Geometry: final body of the model. Coordinates: model frame, mm. A direction names the side the tool comes from. Round coordinates to 2 decimals unless told otherwise and drop trailing zeros. Order: outer loops, then holes, each group sorted by start corner. A loop starts at its lowest first (then second) coordinate and runs counter-clockwise, first axis right, second up. Notation, with made-up numbers: (-9, -27.5) -> (0, -27.5) arc R23 ccw to (0, -3.5) -> close; hole circle Ø5 at (64, 50.25). An arc over 180 degrees is marked (long way). Put each result on its own line as item: value.
```python
from build123d import *


with BuildPart() as part:
    # Sketch1 → Revolve1 (revolve)
    with BuildSketch(Plane.XY, mode=Mode.PRIVATE) as revolve1_sk:
        with BuildLine():
            Line((0, 0), (0, 10))
            Line((0, 10), (15, 10))
            Line((15, 10), (15, 15))
            Line((15, 15), (20, 15))
            ThreePointArc((20, 15), (27.5, 12.990381057), (32.990381057, 7.5))
            Line((32.990381057, 7.5), (35.990381057, 7.5))
            Line((35.990381057, 7.5), (37.490381057, 10))
            Line((37.490381057, 10), (40.490381057, 10))
            Line((40.490381057, 10), (41.990381057, 7.5))
            Line((41.990381057, 7.5), (44.990381057, 7.5))
            Line((44.990381057, 7.5), (46.490381057, 10))
            Line((46.490381057, 10), (49.490381057, 10))
            Line((49.490381057, 10), (50.990381057, 7.5))
            Line((50.990381057, 7.5), (53.990381057, 7.5))
            Line((53.990381057, 7.5), (55.490381057, 10))
            Line((55.490381057, 10), (58.490381057, 10))
            Line((58.490381057, 10), (59.990381057, 7.5))
            Line((59.990381057, 7.5), (62.990381057, 7.5))
            Line((62.990381057, 7.5), (64.490381057, 10))
            Line((64.490381057, 10), (67.490381057, 10))
            ThreePointArc((67.490381057, 10), (70.121555115, 10.607697794), (72.219742949, 12.307692308))
            ThreePointArc((72.219742949, 12.307692308), (94.492324045, 18.911514916), (107.984282589, 0))
            Line((107.984282589, 0), (0, 0))
        make_face()
    revolve(revolve1_sk.sketch.rotate(Axis((0, 0, 0), (1, 0, 0)), 90), axis=Axis((0, 0, 0), (1, 0, 0)))


solid = part.part
```
1. Draft query along X for faces 3 (the face through (0, 0, 0)), 4 (the face through (8, 0, -10)), 5 (the face through (36.084, -2.3, 7.303)). Return one class per face: +X half, -X half, draft (parallel to the pull), parting line (faces both ways), or undercut.
Ans:
face 3: -X half
face 4: draft
face 5: undercut
2. Cut plane B-B on z = 17. Return loops of the section in (x, y).
Ans:
outline: circle Ø21.07 at (87.98, 0)
3. Set-up query: faces 1 (the face through (63.084, -2.3, 7.303)), 2 (the face through (17.54, -12.65, 8.06)). Return all of +Z, -Z, +X, -X, +Y, -Y with unobstructed straight access to the full face (end or side cutting, diameter ignored); none if empty.
Ans:
face 1: none
face 2: -X
4. Material intervals for probe 1 along X at (y, z) = (7.5, 2.5); probe 2 along X at (y, z) = (6, 6); probe 3 along Y at (x, z) = (53.5, 0.5), sorted ascending.
Ans:
probe 1: 0 to 32.75, 36.23 to 41.75, 45.23 to 50.75, 54.23 to 59.75, 63.23 to 106.36
probe 2: 0 to 32.37, 36.58 to 41.4, 45.58 to 50.4, 54.58 to 59.4, 63.58 to 106.1
probe 3: -7.48 to 7.48
5. Contact query for flat-ended pins moving along their axis: P1, Ø3, axis at x = 20.5, z = 8, coming from the +Y side; P2, Ø8, axis at x = 76, z = 8, coming from the -Y side; P3, Ø8, axis at x = 68, y = -13, coming from the -Z side. Output: stop coordinate, or through.
Ans:
P1: y = 13.51
P2: y = -17.08
P3: z = -4.55
6. Cut plane A-A on x = 29. Return loops of the section in (y, z).
Ans:
outline: circle Ø24 at (0, 0)
